Could you check a few things on this model? Use its own coordinates, in mm. Give positions to 0.01 mm unless a question says otherwise; leave off trailing zeros. Write each loop counter-clockwise with the first axis right and the second up, starting at its lowest first coordinate (ties: lowest second). Pieces come first, ordered by that corner, then holes. Notation, with made-up numbers: M 42.5,4 L 62.5,4 A23 ccw 62.5,34 Z; hole C 80.25,-31.5 d3. An arc over 180 degrees is marked long. One line per item, written item: value.
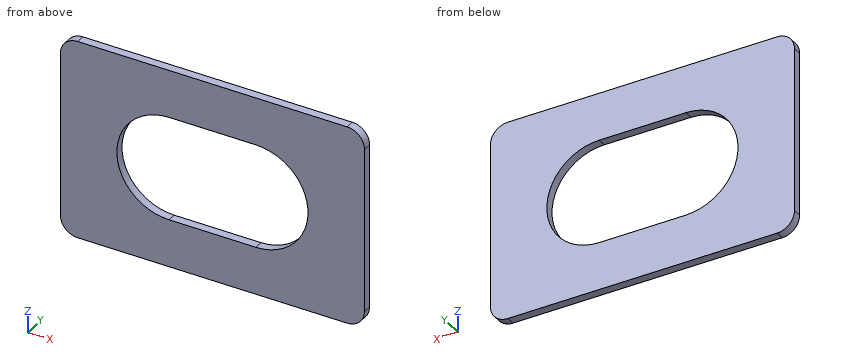
```python
from build123d import *

# Parameters (mm, degrees)
EXTRUDE_1_DEPTH = 1


with BuildPart() as part:
    # Эскиз1 → Бобышка-Вытянуть1 (new body)
    with BuildSketch(Plane(origin=(0, 0, 0), x_dir=(1, 0, 0), z_dir=(0, 1, 0))):
        with BuildLine():
            Line((15.5, -11.5), (-15.5, -11.5))
            ThreePointArc((-15.5, -11.5), (-16.914213562, -10.914213562), (-17.5, -9.5))
            Line((-17.5, -9.5), (-17.5, 9.5))
            ThreePointArc((-17.5, 9.5), (-16.914213562, 10.914213562), (-15.5, 11.5))
            Line((-15.5, 11.5), (15.5, 11.5))
            ThreePointArc((15.5, 11.5), (16.914213562, 10.914213562), (17.5, 9.5))
            Line((17.5, 9.5), (17.5, -9.5))
            ThreePointArc((17.5, -9.5), (16.914213562, -10.914213562), (15.5, -11.5))
        make_face()
        with BuildLine():
            Line((-5, 6), (5, 6))
            ThreePointArc((5, 6), (11, 0), (5, -6))
            Line((5, -6), (-5, -6))
            ThreePointArc((-5, -6), (-11, 0), (-5, 6))
        make_face(mode=Mode.SUBTRACT)
    extrude(amount=EXTRUDE_1_DEPTH)


solid = part.part
```
1) Please list where these lines run through material, in increasing order: L1, parallel to Z at x = -4, y = 0.4; L2, parallel to X at y = 0.8, z = -0.25; L3, parallel to X at y = 0.9, z = -3.25. Write a range as from..to.
Outcome:
L1: z = -11.5..-6, 6..11.5
L2: x = -17.5..-10.99, 10.99..17.5
L3: x = -17.5..-10.04, 10.04..17.5
2) If we section it at B-B, the plane x = -2: Write out the boundary of the cut face in (y, z).
Outcome:
outline: M 0,-11.5 L 1,-11.5 L 1,-6 L 0,-6 Z; M 0,6 L 1,6 L 1,11.5 L 0,11.5 Z
3) If we section it at C-C, the plane y = 0.35: Write out the boundary of the cut face in (x, z), then the cut area to 3 significant figures.
Outcome:
outline: M -17.5,-9.5 A2 ccw -15.5,-11.5 L 15.5,-11.5 A2 ccw 17.5,-9.5 L 17.5,9.5 A2 ccw 15.5,11.5 L -15.5,11.5 A2 ccw -17.5,9.5 Z; hole M -5,-6 L 5,-6 A6 ccw 5,6 L -5,6 A6 ccw Z
area: 568 mm^2
4) If we section it at A-A, the plane z = 0: Write out the boundary of the cut face in (x, y).
Outcome:
outline: M -17.5,0 L -11,0 L -11,1 L -17.5,1 Z; M 11,0 L 17.5,0 L 17.5,1 L 11,1 Z
5) I'm going to push a flat-ended pin straight in: pin 1 (5 mm diameter, centred on x = 10, z = 2.5, fed in from +Y). Where does the tip first touch, or does it pass through?
Outcome:
pin 1: stops at y = 1
